Could you check a few things on this model? Use its own coordinates, in mm. Face numbers are marked on the shaded views. A direction names the side the tool comes from. Give positions to 0.01 mm unless a question says otherwise; leave off trailing zeros. Loops run counter-clockwise (first coordinate to the right, second up) from the corner with the lowest first, then second, coordinate; pieces in that order, holes last. Notation, with made-up numbers: M 33.25,84 L 67.25,84 A21 cw 67.25,93 Z; hole C 59,35.25 d3. An arc over 180 degrees is marked long. Return JSON: item names as keys, results as strings. Group by question number.
1. For pin 1 (4.5 mm diameter, centred on x = -1.5, z = -8, fed in from -Y); pin 2 (12 mm diameter, centred on x = -11, z = 9.5, fed in from +Y); pin 3 (6 mm diameter, centred on y = 1.5, z = -8, fed in from +X); pin 4 (4 mm diameter, centred on y = 7.5, z = -9.5, fed in from +X), each with a flat end and sliding along its axis, tell me the tip position at first contact or that it passes through.
2. Please list where these lines run through material, in increasing order: line 1 (Z direction, x = 0, y = 4.1); line 2 (Z direction, x = 0, y = 14.25); line 3 (Y direction, x = -11.75, z = 1.5).
3. If we section it at C-C (z = -3.75): Write out the boundary of the cut face in (x, y).
4. If we section it at B-B (y = 7.25): Write out the boundary of the cut face in (x, z), plus the area to 3 significant figures.
5. For the marked faces 4, 5 and 6, which set-ups out of +Z, -Z, +X, -X, +Y, -Y let a thin tool reach every point of the face, with its end or its side?
6. If we section it at A-A (x = 0): Write out the boundary of the cut face in (y, z).
7. If we section it at D-D (z = 7.5): Write out the boundary of the cut face in (x, y), plus the area to 3 significant figures.
8. If we mould it in two halves opening along Z, with no side actions, what happens to the marked faces 1, 2 and 3? For each: +Z half, -Z half, draft (parallel to the pull), parting line (faces both ways), or undercut.
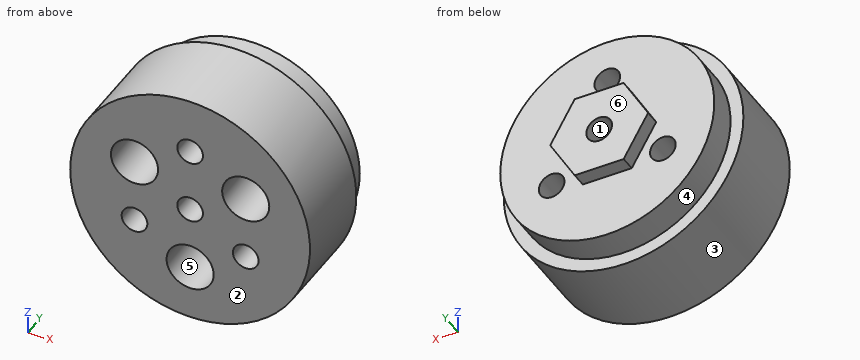
Autodesk Inventor part; units mm, degrees
ref_plane "YZ Plane" through (0, 0, 0) normal (1, 0, 0) x (0, 1, 0)
ref_plane "XZ Plane" through (0, 0, 0) normal (0, 1, 0) x (-1, 0, 0)
ref_plane "XY Plane" through (0, 0, 0) normal (0, 0, 1) x (1, 0, 0)
sketch "Sketch1" plane through (0, 0, 0) normal (0, 1, 0) x (-1, 0, 0)
  circle A0 centre (0, 0) radius 14
  dimension "d0" = 28
extrude "Extrusion1" add sketch "Sketch1" along normal blind 10
sketch "Sketch2" plane through (0, 10, 0) normal (0, 1, 0) x (1, 0, 0)
  circle A0 centre (0, 0) radius 12.5
  dimension "d3" = 25
extrude "Extrusion2" add sketch "Sketch2" along normal blind 3.5
sketch "Sketch3" plane through (0, 0, 0) normal (0, -1, 0) x (1, 0, 0)
  circle A0 centre (0, 0) radius 7.5 construction
  circle A1 centre (0, 0) radius 1.5
  circle A2 centre (0, 7.5) radius 1.5
  circle A3 centre (-6.4952, 3.75) radius 1.5
  circle A4 centre (-6.4952, -3.75) radius 1.5
  circle A5 centre (0, -7.5) radius 1.5
  circle A6 centre (6.4952, -3.75) radius 1.5
  circle A7 centre (6.4952, 3.75) radius 1.5
  dimension "d6" = 15
  dimension "d7" = 3
  dimension "d8" = 3
  dimension "d11" = 360
extrude "Extrusion3" cut sketch "Sketch3" against normal through all contours A1 | A2 | A4 | A6
sketch "Sketch4" plane through (0, 0, 0) normal (0, -1, 0) x (1, 0, 0)
  circle A0 centre (0, 0) radius 7.5
  circle A1 centre (0, -7.5) radius 2.75
  circle A2 centre (0, 0) radius 7.5
  circle A3 centre (6.4952, -3.75) radius 2.75
  circle A4 centre (0, 0) radius 7.5
  circle A5 centre (6.4952, 3.75) radius 2.75
  circle A6 centre (0, 0) radius 7.5
  circle A7 centre (0, 7.5) radius 2.75
  circle A8 centre (0, 0) radius 7.5
  circle A9 centre (-6.4952, 3.75) radius 2.75
  circle A10 centre (0, 0) radius 7.5
  circle A11 centre (-6.4952, -3.75) radius 2.75
  dimension "d15" = 15
  dimension "d16" = 5.5
  dimension "d19" = 360
extrude "Extrusion4" cut sketch "Sketch4" against normal blind 6 contours A5 A0 | A0 A5 | A1 A0 | A0 A1 | A9 A0 | A0 A9
sketch "Sketch5" plane through (0, 13.5, 0) normal (0, 1, 0) x (1, 0, 0)
  line L0 (-2.8579, -4.95) -> (-5.7158, 0)
  line L1 (-5.7158, 0) -> (-2.8579, 4.95)
  line L2 (-2.8579, 4.95) -> (2.8579, 4.95)
  line L3 (2.8579, 4.95) -> (5.7158, 0)
  line L4 (5.7158, 0) -> (2.8579, -4.95)
  line L5 (2.8579, -4.95) -> (-2.8579, -4.95)
  circle A0 centre (0, 0) radius 1.5
  dimension "d23" = 9.9
  dimension "d29" = 3
extrude "Extrusion5" add sketch "Sketch5" along normal blind 1.75
properties part number "Shaft1_Joint1" material "ABS Plastic"
Answer:
{
 "1": {"pin 1": "stops at y = 0", "pin 2": "stops at y = 13.5", "pin 3": "stops at x = 13.08", "pin 4": "stops at x = 11.82"},
 "2": {"line 1": "z = -14 to -10.25, -4.75 to -1.5, 1.5 to 6, 9 to 14", "line 2": "z = -4.95 to -1.5, 1.5 to 4.95", "line 3": "y = 0 to 13.5"},
 "3": {"outline": "M -13.49,0 L -8,0 L -8,13.5 L -11.92,13.5 L -11.92,10 L -13.49,10 Z; M -5,0 L 5,0 L 5,13.5 L 3.55,13.5 L 3.55,15.25 L -3.55,15.25 L -3.55,13.5 L -5,13.5 Z; M 8,0 L 13.49,0 L 13.49,10 L 11.92,10 L 11.92,13.5 L 8,13.5 Z"},
 "4": {"outline": "C 0,0 d28; hole C -6.5,-3.75 d3; hole C 0,0 d3; hole C 0,7.5 d3; hole C 6.5,-3.75 d3", "area": "587 mm²"},
 "5": {"face 4": "+Y", "face 5": "-Y", "face 6": "+Z, -Z, +X, -X, +Y"},
 "6": {"outline": "M 0,-14 L 10,-14 L 10,-12.5 L 13.5,-12.5 L 13.5,-4.95 L 15.25,-4.95 L 15.25,-1.5 L 0,-1.5 L 0,-4.75 L 6,-4.75 L 6,-10.25 L 0,-10.25 Z; M 0,1.5 L 15.25,1.5 L 15.25,4.95 L 13.5,4.95 L 13.5,6 L 0,6 Z; M 0,9 L 13.5,9 L 13.5,12.5 L 10,12.5 L 10,14 L 0,14 Z"},
 "7": {"outline": "M -11.82,0 L -1.5,0 L -1.5,13.5 L -10,13.5 L -10,10 L -11.82,10 Z; M 1.5,0 L 11.82,0 L 11.82,10 L 10,10 L 10,13.5 L 1.5,13.5 Z", "area": "266 mm²"},
 "8": {"face 1": "undercut", "face 2": "draft", "face 3": "parting line"}
}
